Design review of the part built by this model. Coordinates are the model's own, in mm. Coordinates: 2 decimals unless noted, no trailing zeros. Loops run counter-clockwise (first coordinate to the right, second up) from the corner with the lowest first, then second, coordinate; pieces in that order, holes last. Notation, with made-up numbers: (64, 55) - (70, 55) arc R18 cw to (70, 73) - close; hole circle Ø10 at (-16, -39.75). An arc over 180 degrees is marked (long way). Answer in a Markdown table with one row per item. Add a question column.
(1) To check wall thickness, follow L1, parallel to X at y = 2.3, z = -15; L2, parallel to X at y = 1.25, z = -67.5; L3, parallel to Z at x = 26, y = 0.6. State the ranges of each line that lie inside material, in increasing order. Write a range as [from, to].
(2) We need section C-C, the plane z = -27. Write out the cut boundary in (x, y).
(3) We need section B-B, the plane x = 11. Write out the cut boundary in (y, z).
(4) We need section A-A, the plane z = -12.5. Write out the cut boundary in (x, y).
(5) Clearance check with flat-ended pins moving along their axes: pin 1 (0.8 mm diameter, centred on y = 1.5, z = -10, fed in from -X); pin 2 (1.5 mm diameter, centred on y = 1, z = -53.5, fed in from -X); pin 3 (1.3 mm diameter, centred on x = 20.5, y = 1, fed in from -Z). State where each tip first meets the part, or that it passes through.
from build123d import *

# Parameters (mm, degrees)
BOSS_EXTRUDE1_DEPTH = 2.5
SKETCH2_W           = 2.5
SKETCH2_H           = 2.5
CUT_EXTRUDE1_DEPTH  = 10


with BuildPart() as part:
    # Sketch1 → Boss-Extrude1 (new body)
    with BuildSketch(Plane(origin=(0, 0, 0), x_dir=(1, 0, 0), z_dir=(0, 1, 0))):
        Polygon((19.021261999, 44.804158017), (19.332438403, 45.488746105), (20.577144018, 47.604745652), (20.794967501, 48.631627785), (21.527084588, 50.242285376), (21.770981653, 51.392085822), (22.447946599, 52.542926231), (22.447946599, 54.357273616), (21.948192274, 54.857027941), (21.770981653, 56.379920241), (21.990995409, 57.417127949), (21.770981653, 58.340331586), (21.340284184, 60.1475889), (20.68605576, 62.074448432), (19.954791211, 63.47474225), (19.332438403, 65.307720452), (19.332438403, 67.115506175), (19.741207407, 67.810413481), (21.340284184, 67.810413481), (22.992716517, 67.059307875), (24.51836959, 66.161864891), (25.760939094, 64.919295387), (27.687055742, 65.143427014), (29.724933341, 65.143427014), (30.485439327, 65.540580139), (31.279820672, 65.810297182), (32.201793055, 66.437748451), (33.254785535, 68.227835667), (34.276233434, 69.742789054), (35.243443216, 70.709998836), (35.656263686, 71.122819306), (36.913233915, 71.122819306), (37.63391638, 69.742789054), (37.63391638, 66.437748451), (37.423054008, 64.767648146), (37.654974628, 62.774595341), (37.855798717, 62.390038575), (37.855798717, 61.339547521), (38.570896495, 59.97021135), (38.688814239, 57.225826771), (38.50937952, 56.379920241), (38.931857999, 54.607150778), (39.532654393, 51.600225744), (39.660205894, 48.631627785), (39.804568301, 45.271777514), (40.33944819, 44.485828851), (40.577016369, 38.956733507), (40.33944819, 35.114073385), (39.92710204, 34.206911855), (39.92710204, 32.859942326), (37.98561411, 28.148501466), (37.060494228, 20.821243477), (37.11895116, 19.460733181), (36.71985388, 15.068979081), (36.91940252, 11.218958378), (37.185464562, 8.932504932), (37.855798717, 7.947520745), (39.660205894, 7.783546628), (41.232731094, 7.449980677), (41.741559995, 6.702311148), (41.741559995, 5.276917294), (41.050907419, 4.252580704), (40.133275115, 4.033894683), (3.616707841, 4.033894683), (3.616707841, 4.626457176), (3.269950211, 5.647741518), (3.269950211, 6.261397474), (3.269950211, 7.449980677), (3.734735993, 8.139324495), (4.145489026, 10.075731655), (4.493765097, 10.920898955), (3.940112509, 14.699799013), (3.940112509, 17.811459581), (4.189387556, 19.785801077), (4.189387556, 24.971460981), (4.417715683, 28.664663454), (5.09342811, 32.508342262), (6.832899379, 35.465443418), (7.307908954, 36.618157008), (8.257829647, 37.568077701), (8.694357753, 38.627407672), (9.840028976, 39.979843625), (11.786481729, 41.304508301), (13.461509637, 42.616844106), (15.348517574, 43.066547386), (16.554775804, 44.272805615), align=None)
    extrude(amount=BOSS_EXTRUDE1_DEPTH)

    # Sketch2 → Cut-Extrude1 (cut)
    with BuildSketch(Plane.XY.offset(-4.033894683)):
        with Locations((14.819950211, 1.25)):
            Rectangle(SKETCH2_W, SKETCH2_H)
    extrude(amount=-CUT_EXTRUDE1_DEPTH, mode=Mode.SUBTRACT)


solid = part.part
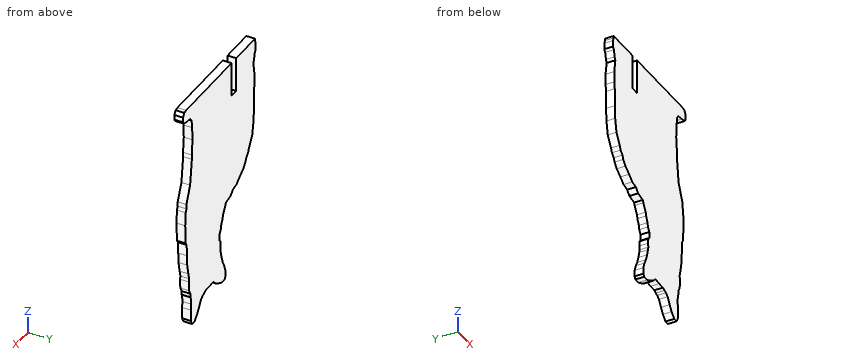
Responses:
| question | item | result |
|---|---|---|
| 1 | L1 | x = [3.94, 36.72] |
| 1 | L2 | x = [19.56, 22.02], [32.83, 37.63] |
| 1 | L3 | z = [-64.95, -4.03] |
| 2 | outline | (4.31, 0) - (37.84, 0) - (37.84, 2.5) - (4.31, 2.5) - close |
| 3 | outline | (0, -40.77) - (2.5, -40.77) - (2.5, -4.03) - (0, -4.03) - close |
| 4 | outline | (4.26, 0) - (13.57, 0) - (13.57, 2.5) - (4.26, 2.5) - close; (16.07, 0) - (36.85, 0) - (36.85, 2.5) - (16.07, 2.5) - close |
| 5 | pin 1 | stops at x = 4.04 |
| 5 | pin 2 | stops at x = 22.45 |
| 5 | pin 3 | stops at z = -67.81 |
